Verification items for this drawing (mm, ordinates from the low corner). A direction names the side the tool comes from. Give positions to 0.01 mm unless a question says otherwise; leave off trailing zeros. Write each loop counter-clockwise with the first axis right and the second up, starting at its lowest first coordinate (ties: lowest second). Pieces come first, ordered by that corner, then holes. Notation, with made-up numbers: M 85.5,65.25 L 101.5,65.25 A20 cw 101.5,89.25 Z; hole C 26.5,-30.75 d1. An arc over 180 degrees is marked long. Write each question's results on one line, items separated by ' | '.
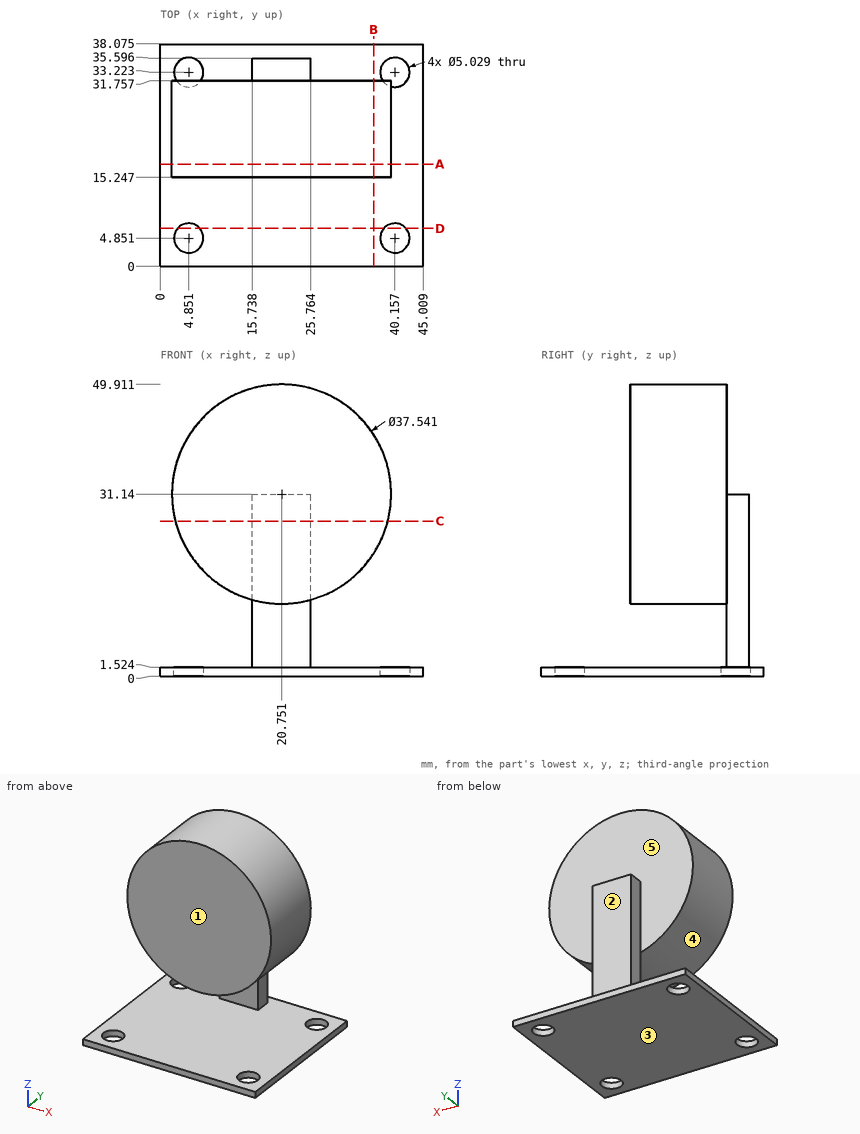
Q1. Section check D-D (y = 6.5). Enter the section's corners in (x, z).
Answer key:
outline: M 0,0 L 2.95,0 L 2.95,1.52 L 0,1.52 Z; M 6.75,0 L 38.26,0 L 38.26,1.52 L 6.75,1.52 Z; M 42.06,0 L 45.01,0 L 45.01,1.52 L 42.06,1.52 Z
Q2. Section check C-C (z = 26.5). Enter the section's corners in (x, y), then the cut area to 3 significant figures.
Answer key:
outline: M 2.56,15.25 L 38.94,15.25 L 38.94,31.76 L 25.76,31.76 L 25.76,35.6 L 15.74,35.6 L 15.74,31.76 L 2.56,31.76 Z | area: 639 mm2
Q3. Section check B-B (x = 36.5). Enter the section's corners in (y, z) (1 decimal).
Answer key:
outline: M 0,0 L 38.1,0 L 38.1,1.5 L 0,1.5 Z; M 15.2,20.9 L 31.8,20.9 L 31.8,41.4 L 15.2,41.4 Z
Q4. Access from +Z, -Z, +X, -X, +Y, -Y to the whole of each face (thin tool, end or side, straight path). Record for the marked faces 1 and 2.
Answer key:
face 1: +Z, +X, -X, -Y | face 2: +Z, +X, -X, +Y
Q5. Section check A-A (y = 17.5). Enter the section's corners in (x, z).
Answer key:
outline: M 0,0 L 45.01,0 L 45.01,1.52 L 0,1.52 Z; C 20.75,31.14 d37.54
Q6. Release check for a two-part mould opening along Z. For the marked faces 3, 4 and 5 record: released by +Z, released by -Z, zero draft, split by the parting line, or undercut.
Answer key:
face 3: released by -Z | face 4: undercut | face 5: zero draft
Q7. Depth check by flat-ended pin: P1, Ø8, axis at y = 20.5, z = 11.5, coming from the +X side; P2, Ø8, axis at x = 37, z = 32.5, coming from the +Y side; P3, Ø11, axis at x = 21, z = 8, coming from the -Y side; P4, Ø2, axis at x = 5.5, y = 15.5, coming from the -Z side. Enter the tip coordinate at first touch or a pass-through.
Answer key:
P1: stops at x = 31.13 | P2: stops at y = 31.76 | P3: stops at y = 15.25 | P4: stops at z = 0
Q8. Material ranges on probe 1 along Y at (x, z) = (4.5, 24); probe 2 along Z at (x, y) = (33, 32.5); probe 3 along X at (y, z) = (32, 5), recorded low to high. Write a range as [from, to].
Answer key:
probe 1: y = [15.25, 31.76] | probe 2: z = [0, 1.52] | probe 3: x = [15.74, 25.76]
